Work out the finished part from the listing and answer in its coordinate system (mm). A direction names the side the tool comes from. Coordinates: 2 decimals unless noted, no trailing zeros. Loops run counter-clockwise (first coordinate to the right, second up) from the corner with the lowest first, then second, coordinate; pieces in that order, holes last. Notation, with made-up numbers: (26, -17.75) -> (78, -17.75) arc R12 ccw to (78, 1.25) -> close; hole circle Ø8 at (67.5, 58.5). An arc over 180 degrees is marked (long way). Answer as CSV lines item,"result".
```python
from build123d import *

# Parameters (mm, degrees)
BOSS_EXTRUDE1_DEPTH = 10
SKETCH2_W           = 30
SKETCH2_H           = 6.318939308
BOSS_EXTRUDE2_DEPTH = 20
FILLET2_R           = 10
FILLET3_R           = 10


with BuildPart() as part:
    # Sketch1 → Boss-Extrude1 (new body)
    with BuildSketch(Plane(origin=(0, 0, 0), x_dir=(1, 0, 0), z_dir=(0, 1, 0))):
        Polygon((0, 0), (0, 50), (150, 76.449047106), (150, -76.449047106), (0, -50), align=None)
    extrude(amount=BOSS_EXTRUDE1_DEPTH)

    # Sketch2 → Boss-Extrude2 (add)
    with BuildSketch(Plane(origin=(0, 10, 0), x_dir=(1, 0, 0), z_dir=(0, 1, 0))):
        with Locations((35, 29.313333891)):
            Rectangle(SKETCH2_W, SKETCH2_H)
    extrude(amount=BOSS_EXTRUDE2_DEPTH)

    # Fillet2
    fillet2_edges = [part.edges().sort_by_distance(p)[0] for p in [
        (20, 30, -29.313333891),
        (50, 30, -29.313333891),
    ]]
    fillet(fillet2_edges, radius=FILLET2_R)

    # Mirror1: part across plane


with BuildPart() as part_1:
    add(part.part)
    add(part.part.mirror(Plane.XY))

    # Fillet3
    fillet3_edges = [part_1.edges().sort_by_distance(p)[0] for p in [
        (150, 5, 76.449047106),
        (150, 5, -76.449047106),
        (0, 5, -50),
        (0, 5, 50),
    ]]
    fillet(fillet3_edges, radius=FILLET3_R)


solid = part_1.part
```
(1) Which of the six approach directions +Z, -Z, +X, -X, +Y, -Y give full straight-line access (tool end or side, diameter ignored) to faces 4 (the face through (35, 20, 32.473)), 5 (the face through (20, 15, -29)), 6 (the face through (35, 20, -32.473))?
Computed values:
face 4,"+Z, +X, -X, +Y"
face 5,"+Z, -Z, -X, +Y"
face 6,"-Z, +X, -X, +Y"
(2) Flat-ended cylindrical pins translate along their axes: pin 1 Ø16 at (x, y) = (40, 21) entering from +Z; pin 2 Ø5 at (y, z) = (14.5, 30) entering from +X; pin 3 Ø1.9 at (y, z) = (13.5, 30.5) entering from -X. Find the tip coordinate at first contact, or state that the pin passes through.
Computed values:
pin 1,"z = 32.47"
pin 2,"x = 50"
pin 3,"x = 20"
(3) Consider line 1 along Z through (x, y) = (27.5, 22.5); line 2 along Y through (x, z) = (55.5, -9); line 3 along Z through (x, y) = (12, 7). Determine where each line is inside the solid, lowest interval first.
Computed values:
line 1,"-32.47 to -26.15, 26.15 to 32.47"
line 2,"0 to 10"
line 3,"-52.12 to 52.12"
(4) For a pull along Z with two mould halves and no side action, classify faces 1 (the face through (35, 20, 26.154)), 2 (the face through (35, 30, 29)), 3 (the face through (74.17, 4.93, 63.08)) as pulls with the +Z half, pulls with the -Z half, needs draft (parallel to the pull), parting line crosses it, or undercut.
Computed values:
face 1,"undercut"
face 2,"needs draft"
face 3,"pulls with the +Z half"
(5) A cutting plane is placed at C-C, the plane y = 5.5. Write down the section's boundary in (x, z), and give its area (3 significant figures).
Computed values:
outline,"(0, -41.61) arc R10 ccw to (8.26, -51.46) -> (138.26, -74.38) arc R10 ccw to (150, -64.53) -> (150, 64.53) arc R10 ccw to (138.26, 74.38) -> (8.26, 51.46) arc R10 ccw to (0, 41.61) -> close"
area,"18,900 mm2"
(6) A cutting plane is placed at B-B, the plane z = 30.5. Write down the section's boundary in (x, y), and give its area (3 significant figures).
Computed values:
outline,"(0, 0) -> (150, 0) -> (150, 10) -> (50, 10) -> (50, 20) arc R10 ccw to (40, 30) -> (30, 30) arc R10 ccw to (20, 20) -> (20, 10) -> (0, 10) -> close"
area,"2,060 mm2"
(7) A cutting plane is placed at D-D, the plane x = 32. Write down the section's boundary in (y, z).
Computed values:
outline,"(0, -55.64) -> (10, -55.64) -> (10, -32.47) -> (30, -32.47) -> (30, -26.15) -> (10, -26.15) -> (10, 26.15) -> (30, 26.15) -> (30, 32.47) -> (10, 32.47) -> (10, 55.64) -> (0, 55.64) -> close"
(8) A cutting plane is placed at A-A, the plane y = 15.75. Write down the section's boundary in (x, z), and give its area (3 significant figures).
Computed values:
outline,"(20, -32.47) -> (50, -32.47) -> (50, -26.15) -> (20, -26.15) -> close; (20, 26.15) -> (50, 26.15) -> (50, 32.47) -> (20, 32.47) -> close"
area,"379 mm2"
